Could you check a few things on this model? Use its own coordinates, in mm. Give positions to 0.01 mm unless a question says otherwise; leave off trailing zeros. Order: outer loops, then holes, each group sorted by start corner. A loop starts at its lowest first (then second) coordinate and runs counter-clockwise, first axis right, second up. Notation, with made-up numbers: (-21.75, 65.25) - (27.25, 65.25) arc R17 ccw to (27.25, 94.25) - close; hole circle Ø6 at (14.5, 32.25). An arc over 180 degrees is marked (long way). Put each result on its own line as item: value.
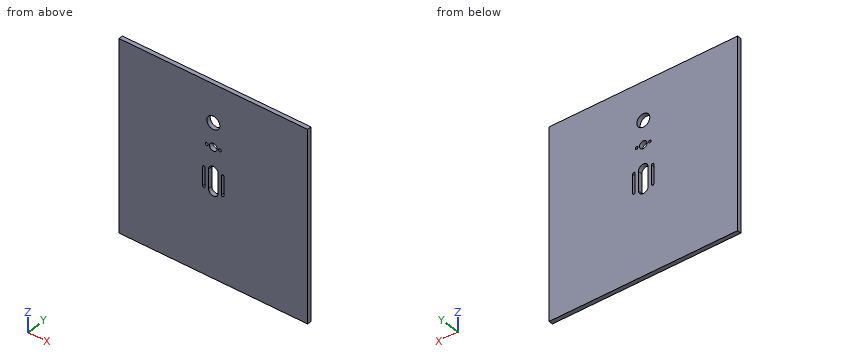
from build123d import *

# Parameters (mm, degrees)
SKETCH1_W           = 254
SKETCH1_H           = 254
BOSS_EXTRUDE1_DEPTH = 5.588
SKETCH2_R           = 8.73125
SKETCH2_R_2         = 5.08
SKETCH2_R_3         = 1.778
CUT_EXTRUDE1_DEPTH  = 180.692030274


with BuildPart() as part:
    # Sketch1 → Boss-Extrude1 (new body)
    with BuildSketch(Plane(origin=(0, 0, 0), x_dir=(1, 0, 0), z_dir=(0, 1, 0))):
        Rectangle(SKETCH1_W, SKETCH1_H)
    extrude(amount=BOSS_EXTRUDE1_DEPTH)

    # Sketch2 → Cut-Extrude1 (cut, through all)
    with BuildSketch(Plane(origin=(0, 5.588, 0), x_dir=(1, 0, 0), z_dir=(0, 1, 0))):
        with Locations(Location((0, -76.2, 0), (0, 0, 270))):
            Circle(SKETCH2_R)
        with Locations(Location((0, -44.45, 0), (0, 0, 270))):
            Circle(SKETCH2_R_2)
        with Locations(Location((-8.89, -44.45, 0), (0, 0, 270))):
            Circle(SKETCH2_R_3)
        with Locations(Location((8.89, -44.45, 0), (0, 0, 270))):
            Circle(SKETCH2_R_3)
        with BuildLine():
            Line((6.5405, 12.7), (6.5405, -12.7))
            ThreePointArc((6.5405, -12.7), (0, -19.2405), (-6.5405, -12.7))
            Line((-6.5405, -12.7), (-6.5405, 12.7))
            ThreePointArc((-6.5405, 12.7), (0, 19.2405), (6.5405, 12.7))
        make_face()
        with BuildLine():
            Line((-11.1125, 12.7), (-11.1125, -12.7))
            ThreePointArc((-11.1125, -12.7), (-12.7, -14.2875), (-14.2875, -12.7))
            Line((-14.2875, -12.7), (-14.2875, 12.7))
            ThreePointArc((-14.2875, 12.7), (-12.7, 14.2875), (-11.1125, 12.7))
        make_face()
        with BuildLine():
            Line((14.2875, 12.7), (14.2875, -12.7))
            ThreePointArc((14.2875, -12.7), (12.7, -14.2875), (11.1125, -12.7))
            Line((11.1125, -12.7), (11.1125, 12.7))
            ThreePointArc((11.1125, 12.7), (12.7, 14.2875), (14.2875, 12.7))
        make_face()
    extrude(amount=-CUT_EXTRUDE1_DEPTH, mode=Mode.SUBTRACT)


solid = part.part
1) If I drill on line 1 (X direction, y = 2.8, z = 44.45); line 2 (Z direction, x = 4, y = 3.85); line 3 (X direction, y = 1.75, z = 49), over which ranges is the centre line in solid material (lowest first)? Write a range as [from, to].
Filled in:
line 1: x = [-127, -10.67], [-7.11, -5.08], [5.08, 7.11], [10.67, 127]
line 2: z = [-127, -17.87], [17.87, 41.32], [47.58, 68.44], [83.96, 127]
line 3: x = [-127, -2.26], [2.26, 127]
2) Suppose I cut it at B-B, the plane x = 0. List the corners of the cut face in (y, z) for me.
Filled in:
outline: (0, -127) - (5.59, -127) - (5.59, -19.24) - (0, -19.24) - close; (0, 19.24) - (5.59, 19.24) - (5.59, 39.37) - (0, 39.37) - close; (0, 49.53) - (5.59, 49.53) - (5.59, 67.47) - (0, 67.47) - close; (0, 84.93) - (5.59, 84.93) - (5.59, 127) - (0, 127) - close
3) I'm going to push a flat-ended pin straight in: pin 1 (15.5 mm diameter, centred on x = 0, z = 76.2, fed in from +Y). Where does the tip first touch, or does it pass through?
Filled in:
pin 1: passes through
4) Suppose I cut it at C-C, the plane z = 76.2. List the corners of the cut face in (x, y) for me.
Filled in:
outline: (-127, 0) - (-8.73, 0) - (-8.73, 5.59) - (-127, 5.59) - close; (8.73, 0) - (127, 0) - (127, 5.59) - (8.73, 5.59) - close
5) Suppose I cut it at D-D, the plane y = 2.3. State how many separate pieces and enclosed holes the cut face has, and give its area (3 significant figures).
Filled in:
separate pieces: 1
enclosed holes: 7
area: 63,500 mm^2
6) Suppose I cut it at A-A, the plane z = -4. List the corners of the cut face in (x, y) for me.
Filled in:
outline: (-127, 0) - (-14.29, 0) - (-14.29, 5.59) - (-127, 5.59) - close; (-11.11, 0) - (-6.54, 0) - (-6.54, 5.59) - (-11.11, 5.59) - close; (6.54, 0) - (11.11, 0) - (11.11, 5.59) - (6.54, 5.59) - close; (14.29, 0) - (127, 0) - (127, 5.59) - (14.29, 5.59) - close
